Could you check a few things on this model? Use its own coordinates, in mm. A direction names the side the tool comes from. Coordinates: 2 decimals unless noted, no trailing zeros. Order: outer loops, then holes, each group sorted by start corner. A loop starts at its lowest first (then second) coordinate and runs counter-clockwise, first axis right, second up.
Autodesk Fusion 360 part; units mm, degrees
sketch "Sketch4" plane through (0, 0, 0) normal (0, 0, 1) x (-1, 0, 0)
  circle A0 centre (0, 0) radius 15.7
  arc A1 (6.1849, 14.4304) -> (7.9716, 12.1501) centre (10.6805, 16.1127) ccw
  arc A2 (6.1849, 14.4304) -> (-5.1632, 14.8267) centre (0, 0) ccw
  arc A3 (-7.1047, 12.6765) -> (-5.1632, 14.8267) centre (-9.5305, 16.8184) ccw
  arc A4 (-7.1047, 12.6765) -> (-12.1501, 7.9716) centre (0.8594, -0.9216) ccw
  arc A5 (-14.4304, 6.1849) -> (-12.1501, 7.9716) centre (-16.1127, 10.6805) ccw
  arc A6 (-14.4304, 6.1849) -> (-14.8267, -5.1632) centre (0, 0) ccw
  arc A7 (-12.6765, -7.1047) -> (-14.8267, -5.1632) centre (-16.8184, -9.5305) ccw
  arc A8 (-12.6765, -7.1047) -> (-7.9716, -12.1501) centre (0.9216, 0.8594) ccw
  arc A9 (-6.1849, -14.4304) -> (-7.9716, -12.1501) centre (-10.6805, -16.1127) ccw
  arc A10 (-6.1849, -14.4304) -> (5.1632, -14.8267) centre (0, 0) ccw
  arc A11 (7.1047, -12.6765) -> (5.1632, -14.8267) centre (9.5305, -16.8184) ccw
  arc A12 (7.1047, -12.6765) -> (12.1501, -7.9716) centre (-0.8594, 0.9216) ccw
  arc A13 (14.4304, -6.1849) -> (12.1501, -7.9716) centre (16.1127, -10.6805) ccw
  arc A14 (14.4304, -6.1849) -> (14.8267, 5.1632) centre (0, 0) ccw
  arc A15 (12.6765, 7.1047) -> (14.8267, 5.1632) centre (16.8184, 9.5305) ccw
  arc A16 (12.6765, 7.1047) -> (7.9716, 12.1501) centre (-0.9216, -0.8594) ccw
  dimension "d11" = 31.4
sketch "Sketch1" plane through (0, 0, 0) normal (0, 1, 0) x (1, 0, 0)
  line L0 (0, 0) -> (0, -17.25)
  line L1 (0, 0) -> (15.5, 0)
  line L2 (15.5, 0) -> (15.5, -7)
  line L3 (15.5, -7) -> (14.23, -13.605)
  line L4 (14.23, -13.605) -> (14.23, -17.25)
  line L5 (14.23, -17.25) -> (0, -17.25)
  dimension "d1" = 15.5
  dimension "d2" = 14.23
  dimension "d3" = 3.645
  dimension "d4" = 7
  dimension "d5" = 17.25
revolve "Revolve1" add sketch "Sketch1" angle 360 about axis through (0, 0, 1.75) along (0, 0, 1)
sketch "Sketch2" plane through (0, 0, 0) normal (0, 0, -1) x (1, 0, 0)
  circle A0 centre (0, 0) radius 15.5
  circle A1 centre (0, 0) radius 9.085
  circle A2 centre (0, 0) radius 12.5
  line L0 (0, 0) -> (26.4938, 0) construction
  line L1 (0, 0) -> (0, 20.2896) construction
  circle A3 centre (9.5305, 16.8184) radius 5
  circle A4 centre (16.1127, 10.6805) radius 5
  line L2 (0, 0) -> (18.26, 19.5815) construction
  line L3 (9.5305, 16.8184) -> (16.1127, 10.6805)
  arc A5 (11.9849, 7.8588) -> (7.0036, 12.504) centre (-0.8594, -0.9216) ccw
  line L4 (12.9405, 20.4752) -> (19.5227, 14.3372)
  dimension "d7" = 18.17
  dimension "d8" = 25
  dimension "d12" = 10
  dimension "d13" = 9
  dimension "d14" = 18.8
  dimension "d24" = 47
extrude "Extrude1" cut sketch "Sketch2" against normal blind 2.85 contours A2
extrude "Extrude2" cut sketch "Sketch2" against normal blind 22 contours A0 A4 | A0 A3 A4 | A0 A3 A4 | A0 A3 | A0 A3 A4 A5 | A0 A3 A4 | A3 A4 L4 | A3 A4 L3 | A3 A4 L3 picked at (10.0669, 10.6715)
pattern_circular "C-Pattern1" count 4 over 360 about axis through (0, 0, 1.75) along (0, 0, 1) of "Extrude2"
sketch "Sketch3" plane through (0, 0, 17.25) normal (0, 0, 1) x (-1, 0, 0)
  circle A0 centre (0, 0) radius 13.175
  circle A1 centre (0, 0) radius 14.23
  dimension "d19" = 26.35
extrude "Extrude4" [suppressed]
equation "d1 = ( 31 / 2 ) * 1 mm"
equation "d2 = ( 28.46 / 2 ) * 1 mm"
Item 1: Which directions (+Z, -Z, +X, -X, +Y, -Y) give clear straight access to the entire face, cutting with the end or side of a thin tool? Please do faces 5 (the face through (-3.085, -13.892, 15.453)), 6 (the face through (-1.18, -9.01, 1.41)), 7 (the face through (-9.79, 10.42, 6.53)).
Item 2: Thinking about a two-plate mould opening in Y: for faces 1 (the face through (-12.979, 6.785, 4.994)), 2 (the face through (0.9, 9.2, 2.85)), 3 (the face through (-6.785, -12.979, 4.994)), 4 (the face through (0, -13, 0)), which applies, +Y half, -Y half, draft (parallel to the pull), parting line (faces both ways), or undercut?
Item 3: I need wall thicknesses on line 1 (X direction, y = 0, z = 2.25) (3 decimals); line 2 (Z direction, x = -6, y = 9.5). Which ranges of each line are inside material? Lowest first, please.
Item 4: Suppose I cut it at A-A (y = 0). List the corners of the cut face in (x, z) for me (3 decimals), and give its area (3 significant figures).
Item 5: Suppose I cut it at C-C (z = 16.25). List the corners of the cut face in (x, y) for me.
Item 6: For pin 1 Ø5 at (x, z) = (11, 9) entering from +Y; pin 2 Ø10 at (x, z) = (2, 5) entering from -Y; pin 3 Ø1.5 at (y, z) = (-5.5, 14) entering from +X; pin 4 Ø1 at (y, z) = (-8, 8.5) entering from -X, each with a flat end and sliding along its axis, tell me the tip position at first contact or that it passes through.
Geometry results:
1. face 5: +Z
1. face 6: -Z
1. face 7: +Z, -Z, -X, +Y
2. face 1: +Y half
2. face 2: undercut
2. face 3: -Y half
2. face 4: draft
3. line 1: x = -15.5 to -12.5, -9.085 to 9.085, 12.5 to 15.5
3. line 2: z = 2.85 to 17.25
4. outline: (-15.5, 0) - (-12.5, 0) - (-12.5, 2.85) - (-9.085, 2.85) - (-9.085, 0) - (9.085, 0) - (9.085, 2.85) - (12.5, 2.85) - (12.5, 0) - (15.5, 0) - (15.5, 7) - (14.23, 13.605) - (14.23, 17.25) - (-14.23, 17.25) - (-14.23, 13.605) - (-15.5, 7) - close
4. area: 498 mm2
5. outline: circle Ø28.46 at (0, 0)
6. pin 1: stops at y = 11.52
6. pin 2: stops at y = -15.5
6. pin 3: stops at x = 13.41
6. pin 4: stops at x = -12.2
